from build123d import *

# Parameters (mm, degrees)
F2_R    = 0.381
F3_SIZE = 0.381


with BuildPart() as f1:
    # F0 (on Front) → F1 (revolve)
    with BuildSketch(Plane.XZ):
        Polygon((-26, 0), (-17.145, 0), (-17.145, 6.35), (-32.35, 6.35), (-32.35, -6.35), (-42.35, -6.35), (-42.35, -73.775001), (-61.4, -73.775001), (-61.4, -80.125001), (-36, -80.125001), (-36, -12.7), (-26, -12.7), align=None)
    revolve(axis=Axis((0, 0, -27.375497), (0, 0, -1)))

    # F2
    f2_edges = [f1.edges().sort_by_distance(p)[0] for p in [
        (32.35, 0, -6.35),
        (42.35, 0, -73.775001),
        (36, 0, -12.7),
        (26, 0, 0),
    ]]
    fillet(f2_edges, radius=F2_R)

    # F3
    f3_edges = [f1.edges().sort_by_distance(p)[0] for p in [
        (32.35, 0, 6.35),
        (17.145, 0, 6.35),
        (42.35, 0, -6.35),
        (61.4, 0, -73.775001),
        (61.4, 0, -80.125001),
        (36, 0, -80.125001),
        (26, 0, -12.7),
        (17.145, 0, 0),
    ]]
    chamfer(f3_edges, length=F3_SIZE)


solid = f1.part
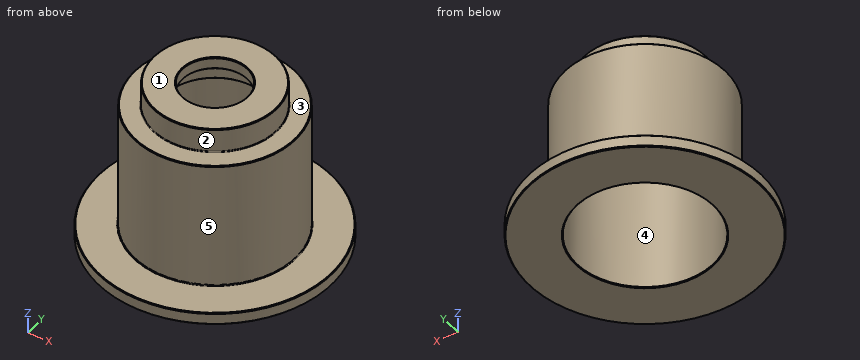
Here's how the part is built. I have some questions about the finished solid (model axes, mm). Face numbers are marked on the shaded views. A direction names the side the tool comes from. Round coordinates to 2 decimals unless told otherwise and drop trailing zeros. Loops run counter-clockwise (first coordinate to the right, second up) from the corner with the lowest first, then second, coordinate; pieces in that order, holes last. Notation, with made-up numbers: (28, 16) -> (36, 16) arc R30 cw to (36, 42) -> close; hole circle Ø5 at (26.25, -12.75). An arc over 180 degrees is marked (long way). Write each question's results on one line, items separated by ' | '.
(1) For the marked faces 1 and 2, which set-ups out of +Z, -Z, +X, -X, +Y, -Y let a thin tool reach every point of the face, with its end or its side?
Worked answers:
face 1: +Z, +X, -X, +Y, -Y | face 2: +Z
(2) If I drill on L1, parallel to Y at x = 0, z = -3.25; L2, parallel to Y at x = 0, z = -10; L3, parallel to Z at x = 12.5, y = -47 (3 decimals), over which ranges is the centre line in solid material (lowest first)?
Worked answers:
L1: -32.35 to -26, 26 to 32.35 | L2: -42.35 to -26, 26 to 42.35 | L3: -80.125 to -73.775
(3) If we section it at B-B, the plane z = -71: List the corners of the cut face in (x, y) for me, then the cut area to 3 significant figures.
Worked answers:
outline: circle Ø84.7 at (0, 0); hole circle Ø72 at (0, 0) | area: 1,560 mm2
(4) For P1, Ø4, axis at y = -2, z = -40.5, coming from the -X side; P2, Ø3, axis at y = 27.5, z = -30.5, coming from the -X side; P3, Ø8, axis at x = -25.5, z = -57, coming from the +Y side, each with a flat end and sliding along its axis, tell me the tip position at first contact or that it passes through.
Worked answers:
P1: x = -42.35 | P2: x = -33.43 | P3: y = 36.49
(5) We'd pull the mould along Y, two halves only. Please class the marked faces 3, 4 and 5: released by +Y, released by -Y, zero draft, split by the parting line, or undercut.
Worked answers:
face 3: zero draft | face 4: undercut | face 5: split by the parting line
(6) If we section it at A-A, the plane z = -2: List the corners of the cut face in (x, y) for me.
Worked answers:
outline: circle Ø64.7 at (0, 0); hole circle Ø52 at (0, 0)
